```python
from build123d import *

# Parameters (mm, degrees)
SKETCH1_R                   = 35
BOSS_EXTRUDE1_DEPTH         = 10
SKETCH2_R                   = 23
BOSS_EXTRUDE2_DEPTH         = 7
BOSS_EXTRUDE3_DEPTH         = 4
SKETCH5_R                   = 1.5
CUT_EXTRUDE1_DEPTH          = 4
FILLET1_R                   = 2
FILLET1_OF_MIRROR1_R        = 2
SKETCH6_W                   = 6
SKETCH6_H                   = 2
BOSS_EXTRUDE4_DEPTH         = 10
FILLET2_RADIUS              = 1
FILLET2_LENGTH              = 10
FILLET2_OF_MIRROR2_2_RADIUS = 1
FILLET2_OF_MIRROR2_2_LENGTH = 10
SKETCH7_R                   = 15
CUT_EXTRUDE2_DEPTH          = 10


with BuildPart() as part:
    # Sketch1 → Boss-Extrude1 (new body)
    with BuildSketch(Plane(origin=(0, 0, 0), x_dir=(1, 0, 0), z_dir=(0, 1, 0))):
        with Locations(Location((0, 0, 0), (0, 0, 270))):
            Circle(SKETCH1_R)
    extrude(amount=BOSS_EXTRUDE1_DEPTH)

    # Sketch2 → Boss-Extrude2 (add)
    with BuildSketch(Plane(origin=(0, 10, 0), x_dir=(1, 0, 0), z_dir=(0, 1, 0))):
        with Locations(Location((0, 0, 0), (0, 0, 270))):
            Circle(SKETCH2_R)
    extrude(amount=BOSS_EXTRUDE2_DEPTH)

    # Sketch4 → Boss-Extrude3 (add)
    with BuildSketch(Plane(origin=(13, 0, 0), x_dir=(0, 0, -1), z_dir=(1, 0, 0))):
        Polygon((35, 17), (-35, 17), (-44.194, 24.714682009), (-44.194, 29.714682009), (-27.952, 43.343338219), (27.952, 43.343338219), (44.194, 29.714682009), (44.194, 24.714682009), align=None)
    boss_extrude3 = extrude(amount=-BOSS_EXTRUDE3_DEPTH)

    # Sketch5 → Cut-Extrude1 (cut)
    with BuildSketch(Plane(origin=(13, 0, 0), x_dir=(0, 0, -1), z_dir=(1, 0, 0))):
        with Locations((-41.194, 27.214682009)):
            Circle(SKETCH5_R)
        with Locations(Location((41.194, 27.214682009, 0), (0, 0, 180))):
            Circle(SKETCH5_R)
    cut_extrude1 = extrude(amount=-CUT_EXTRUDE1_DEPTH, mode=Mode.SUBTRACT)

    # Fillet1
    fillet1_edges = [part.edges().sort_by_distance(p)[0] for p in [
        (11, 43.343338219, 27.952),
        (11, 43.343338219, -27.952),
        (11, 29.714682009, -44.194),
        (11, 24.714682009, -44.194),
        (11, 24.714682009, 44.194),
        (11, 29.714682009, 44.194),
    ]]
    fillet(fillet1_edges, radius=FILLET1_R)

    # Mirror1: Boss-Extrude3, Cut-Extrude1 across plane
    add(boss_extrude3.mirror(Plane(origin=(0, 0, 0), x_dir=(0, 0, 1), z_dir=(1, 0, 0))))
    add(cut_extrude1.mirror(Plane(origin=(0, 0, 0), x_dir=(0, 0, 1), z_dir=(1, 0, 0))), mode=Mode.SUBTRACT)

    # Fillet1 of Mirror1
    fillet1_of_mirror1_edges = [part.edges().sort_by_distance(p)[0] for p in [
        (-11, 43.343338219, 27.952),
        (-11, 43.343338219, -27.952),
        (-11, 29.714682009, -44.194),
        (-11, 24.714682009, -44.194),
        (-11, 24.714682009, 44.194),
        (-11, 29.714682009, 44.194),
    ]]
    fillet(fillet1_of_mirror1_edges, radius=FILLET1_OF_MIRROR1_R)

    # Sketch6 → Boss-Extrude4 (add)
    with BuildSketch(Plane(origin=(0, 17, 0), x_dir=(1, 0, 0), z_dir=(0, 1, 0))):
        with Locations((-16, 0)):
            Rectangle(SKETCH6_W, SKETCH6_H)
    boss_extrude4 = extrude(amount=BOSS_EXTRUDE4_DEPTH)

    # Fillet2: full round fillet: the end face becomes a half cylinder, R = half its width
    fillet2_face = Plane((-19, 22, 0), x_dir=(0, -1, 0), z_dir=(-1, 0, 0))  # on the end face: x along it, z out of the body
    fillet2_slab = fillet2_face.offset(-FILLET2_RADIUS / 2) * Box(FILLET2_LENGTH, 2 * FILLET2_RADIUS, FILLET2_RADIUS, mode=Mode.PRIVATE)  # the body's end, R deep
    fillet2_round = Plane((-18, 22, 0), x_dir=(-1, 0, 0), z_dir=(0, -1, 0)) * Cylinder(FILLET2_RADIUS, FILLET2_LENGTH, mode=Mode.PRIVATE)  # its axis R under the face
    add(fillet2_slab - fillet2_round, mode=Mode.SUBTRACT)

    # Mirror2: Boss-Extrude4 across plane
    add(boss_extrude4.mirror(Plane(origin=(0, 0, 0), x_dir=(0, 0, 1), z_dir=(1, 0, 0))))

    # Fillet2 of Mirror2 2: full round fillet: the end face becomes a half cylinder, R = half its width
    fillet2_of_mirror2_2_face = Plane((19, 22, 0), x_dir=(0, -1, 0), z_dir=(1, 0, 0))  # on the end face: x along it, z out of the body
    fillet2_of_mirror2_2_slab = fillet2_of_mirror2_2_face.offset(-FILLET2_OF_MIRROR2_2_RADIUS / 2) * Box(FILLET2_OF_MIRROR2_2_LENGTH, 2 * FILLET2_OF_MIRROR2_2_RADIUS, FILLET2_OF_MIRROR2_2_RADIUS, mode=Mode.PRIVATE)  # the body's end, R deep
    fillet2_of_mirror2_2_round = Plane((18, 22, 0), x_dir=(1, 0, 0), z_dir=(0, -1, 0)) * Cylinder(FILLET2_OF_MIRROR2_2_RADIUS, FILLET2_OF_MIRROR2_2_LENGTH, mode=Mode.PRIVATE)  # its axis R under the face
    add(fillet2_of_mirror2_2_slab - fillet2_of_mirror2_2_round, mode=Mode.SUBTRACT)

    # Sketch7 → Cut-Extrude2 (cut)
    with BuildSketch(Plane.XZ):
        with Locations(Location((0, 0, 0), (0, 0, 270))):
            Circle(SKETCH7_R)
    extrude(amount=-CUT_EXTRUDE2_DEPTH, mode=Mode.SUBTRACT)


solid = part.part
```
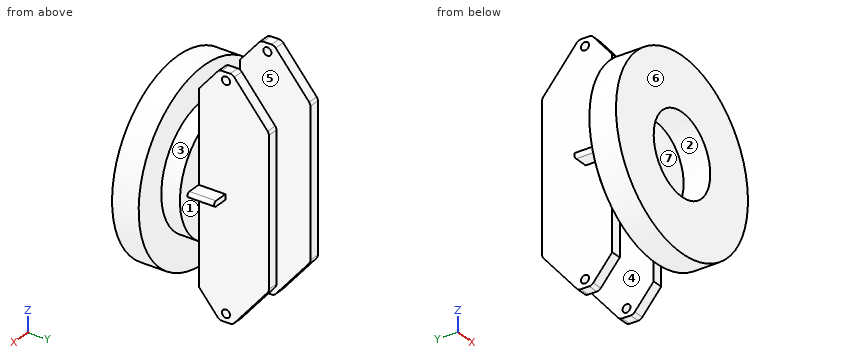
Verification items for the finished model (mm, model axes). Face numbers are marked on the shaded views. A direction names the side the tool comes from. Coordinates: 2 decimals unless noted, no trailing zeros. Write each loop counter-clockwise with the first axis right and the second up, starting at its lowest first coordinate (ties: lowest second). Pieces come first, ordered by that corner, then holes. Notation, with made-up numbers: (28.25, 41.25) - (52.25, 41.25) arc R18 ccw to (52.25, 69.25) - close; hole circle Ø6 at (66.25, 79.5). An arc over 180 degrees is marked (long way). One line per question, with ' | ' between items. Start each with the question number.
1. Section check A-A (y = 18). Enter the section's corners in (x, z).
2. Access from +Z, -Z, +X, -X, +Y, -Y to the whole of each face (thin tool, end or side, straight path). Record for the marked faces 5, 6 and 7.
3. Section check D-D (y = 39). Enter the section's corners in (x, z), plus the area to 3 significant figures.
4. Material ranges on line 1 along X through (y, z) = (24.5, 32); line 2 along X through (y, z) = (7.5, 0); line 3 along Y through (x, z) = (4.5, -28), recorded low to high.
5. Section check C-C (x = -6.5). Enter the section's corners in (y, z), plus the area to 3 significant figures.
6. Draft check along X on the marked faces 1, 2, 3 and 4. Enter one of: released by +X, released by -X, zero draft, split by the parting line, or undercut.
7. Gauge pin test, flat ends, axial feed: P1, Ø4, axis at y = 27.21, z = -41.19, coming from the +X side; P2, Ø2.5, axis at x = -15.5, y = 21, coming from the -Z side; P3, Ø6, axis at y = 36.5, z = -18.5, coming from the -X side; P4, Ø1.8, axis at y = 27.21, z = 41.19, coming from the -X side. Record the tip position at first contact, or that the pin passes through.
8. Section check B-B (z = 0). Enter the section's corners in (x, y).
Computed values:
1) outline: (-18, -1) - (-13, -1) - (-13, -36.19) - (-9, -36.19) - (-9, 36.19) - (-13, 36.19) - (-13, 1) - (-18, 1) arc R1 ccw to start; (9, -36.19) - (13, -36.19) - (13, -1) - (18, -1) arc R1 ccw to (18, 1) - (13, 1) - (13, 36.19) - (9, 36.19) - close
2) face 5: +Z, -Z, +Y | face 6: +Z, -Z, +X, -X, -Y | face 7: -Y
3) outline: (-13, -33.13) - (-9, -33.13) - (-9, 33.13) - (-13, 33.13) - close; (9, -33.13) - (13, -33.13) - (13, 33.13) - (9, 33.13) - close | area: 530 mm²
4) line 1: -13 to -9, 9 to 13 | line 2: -35 to -15, 15 to 35 | line 3: 0 to 10
5) outline: (0, -34.39) - (10, -34.39) - (10, -22.06) - (17, -22.06) - (17, 22.06) - (10, 22.06) - (10, 34.39) - (0, 34.39) - (0, 13.52) - (10, 13.52) - (10, -13.52) - (0, -13.52) - close | area: 726 mm²
6) face 1: zero draft | face 2: undercut | face 3: split by the parting line | face 4: undercut
7) P1: x = 13 | P2: z = -1 | P3: x = -13 | P4: through
8) outline: (-35, 0) - (-15, 0) - (-15, 10) - (15, 10) - (15, 0) - (35, 0) - (35, 10) - (23, 10) - (23, 17) - (19, 17) - (19, 27) - (13, 27) - (13, 43.34) - (9, 43.34) - (9, 17) - (-9, 17) - (-9, 43.34) - (-13, 43.34) - (-13, 27) - (-19, 27) - (-19, 17) - (-23, 17) - (-23, 10) - (-35, 10) - close
